Model file for the job. Use its own axes, mm. Face numbers are marked on the shaded views. A direction names the side the tool comes from. Give positions to 0.01 mm unless a question says otherwise; leave off trailing zeros. Write each loop counter-clockwise with the first axis right and the second up, starting at its lowest first coordinate (ties: lowest second). Pieces come first, ordered by that corner, then holes.
```python
from build123d import *

# Parameters (mm, degrees)
F0_W          = 23
F0_H          = 17.5
F1_DEPTH      = 9
F2_T          = -1.2
F3_R          = 5.7
F4_DEPTH      = 3
F3_R_2        = 6.7
F5_DEPTH      = 7.5
F6_W          = 6
F6_H          = 2.3
F6_W_2        = 3.5
F6_H_2        = 3.5
F7_DEPTH      = 4
F8_DEPTH      = 6
F10_DEPTH     = 30
F11_T1_DEPTH  = 19
F11_T3_DEPTH  = 26.5
F11_T5_DEPTH  = 12
F11_T7_DEPTH  = 28.3038475773
F11_S11_W     = 2
F11_S11_H     = 2
F11_T12_DEPTH = 2
F11_S17_W     = 2
F11_S17_H     = 2
F11_T18_DEPTH = 2


# Not quite as in the source:
# - a fillet or chamfer that OpenCascade refuses, or shapes differently, is made with other operations: its cross-section is extruded or revolved along the edge and cut away or added


with BuildPart() as f1:
    # F0 (on Front) → F1 (new body)
    with BuildSketch(Plane.XZ):
        Rectangle(F0_W, F0_H)
    extrude(amount=F1_DEPTH)

    # F2
    f2_openings = [f1.faces().sort_by_distance(p)[0] for p in [
        (0, -9, 0),
    ]]
    offset(amount=F2_T, openings=f2_openings)

    # F3 (on face) → F4 (cut)
    with BuildSketch(Plane(origin=(0, 0, 0), x_dir=(-1, 0, 0), z_dir=(0, 1, 0))):
        Circle(F3_R)
    extrude(amount=-F4_DEPTH, mode=Mode.SUBTRACT)

    # F3 (on face) → F5 (join)
    with BuildSketch(Plane(origin=(0, 0, 0), x_dir=(-1, 0, 0), z_dir=(0, 1, 0))):
        Circle(F3_R_2)
        Circle(F3_R, mode=Mode.SUBTRACT)
    extrude(amount=F5_DEPTH)

    # F6 (on face) → F7 (cut)
    with BuildSketch(Plane.XY.offset(8.75)):
        with Locations((1.5, -7.85)):
            Rectangle(F6_W, F6_H)
        with Locations((-5.75, -7.25)):
            Rectangle(F6_W_2, F6_H_2)
    extrude(amount=-F7_DEPTH, mode=Mode.SUBTRACT)

    # F8 (add): a face of the model
    f8_faces = [f1.faces().sort_by_distance(p)[0] for p in [
        (0, -4.5, -8.75),
    ]]
    extrude(f8_faces, amount=F8_DEPTH)

    # F9 (on face) → F10 (cut)
    with BuildSketch(Plane.YZ.offset(11.5)):
        Polygon((-9, -14.75), (0, -14.75), (-9, -9.5538475773), align=None)
    extrude(amount=-F10_DEPTH, mode=Mode.SUBTRACT)

    # F11: fillet of radius 2 on 7 edges, made by hand

    # F11_s2 → F11_t1 (cut)
    with BuildSketch(Plane.YZ.offset(-9.5)):
        with BuildLine():
            ThreePointArc((0, 6.75), (-0.5857864376, 8.1642135624), (-2, 8.75))
            Line((-2, 8.75), (0, 8.75))
            Line((0, 8.75), (0, 6.75))
        make_face()
    extrude(amount=F11_T1_DEPTH, mode=Mode.SUBTRACT)

    # F11_s4 → F11_t3 (cut)
    with BuildSketch(Plane.XY.offset(-19.75)):
        with BuildLine():
            ThreePointArc((-11.5, -2), (-10.9142135624, -0.5857864376), (-9.5, 0))
            Line((-9.5, 0), (-11.5, 0))
            Line((-11.5, 0), (-11.5, -2))
        make_face()
        with BuildLine():
            ThreePointArc((9.5, 0), (10.9142135624, -0.5857864376), (11.5, -2))
            Line((11.5, -2), (11.5, 0))
            Line((11.5, 0), (9.5, 0))
        make_face()
    extrude(amount=F11_T3_DEPTH, mode=Mode.SUBTRACT)

    # F11_s6 → F11_t5 (cut)
    with BuildSketch(Plane.XZ.offset(2)):
        with BuildLine():
            ThreePointArc((9.5, 8.75), (10.9142135624, 8.1642135624), (11.5, 6.75))
            Line((11.5, 6.75), (11.5, 8.75))
            Line((11.5, 8.75), (9.5, 8.75))
        make_face()
        with BuildLine():
            ThreePointArc((-11.5, 6.75), (-10.9142135624, 8.1642135624), (-9.5, 8.75))
            Line((-9.5, 8.75), (-11.5, 8.75))
            Line((-11.5, 8.75), (-11.5, 6.75))
        make_face()
    extrude(amount=F11_T5_DEPTH, mode=Mode.SUBTRACT)

    # F11_s8 → F11_t7 (cut)
    with BuildSketch(Plane.XY.offset(-14.5538475773)):
        with BuildLine():
            ThreePointArc((-11.5, -7), (-10.9142135624, -8.4142135624), (-9.5, -9))
            Line((-9.5, -9), (-11.5, -9))
            Line((-11.5, -9), (-11.5, -7))
        make_face()
        with BuildLine():
            ThreePointArc((9.5, -9), (10.9142135624, -8.4142135624), (11.5, -7))
            Line((11.5, -7), (11.5, -9))
            Line((11.5, -9), (9.5, -9))
        make_face()
    extrude(amount=F11_T7_DEPTH, mode=Mode.SUBTRACT)


with BuildPart() as f11_tool10:
    # F11_s11 → F11_t12 (new body)
    with BuildSketch(Plane.XZ.offset(2)):
        with Locations((10.5, 7.75)):
            Rectangle(F11_S11_W, F11_S11_H)
    extrude(amount=-F11_T12_DEPTH)

    # F11_s13 → F11_t14 (revolve, cut)
    with BuildSketch(Plane(origin=(9.5, -2, 6.75), x_dir=(-0.7071067812, 0, -0.7071067812), z_dir=(0.7071067812, 0, -0.7071067812))):
        with BuildLine():
            ThreePointArc((0, -2), (2, 0), (0, 2))
            Line((0, 2), (0, -2))
        make_face()
    revolve(axis=Axis((9.5, -2, 6.75), (0, 1, 0)), mode=Mode.SUBTRACT)


with BuildPart() as f1_1:
    add(f1.part)

    # F11_t9: cut F11_tool10
    add(f11_tool10.part, mode=Mode.SUBTRACT)


with BuildPart() as f11_tool16:
    # F11_s17 → F11_t18 (new body)
    with BuildSketch(Plane.YZ.offset(-9.5)):
        with Locations((-1, 7.75)):
            Rectangle(F11_S17_W, F11_S17_H)
    extrude(amount=-F11_T18_DEPTH)

    # F11_s19 → F11_t20 (revolve, cut)
    with BuildSketch(Plane(origin=(-9.5, -2, 6.75), x_dir=(0, -0.7071067812, -0.7071067812), z_dir=(0, 0.7071067812, -0.7071067812))):
        with BuildLine():
            ThreePointArc((0, -2), (2, 0), (0, 2))
            Line((0, 2), (0, -2))
        make_face()
    revolve(axis=Axis((-9.5, -2, 6.75), (-1, 0, 0)), mode=Mode.SUBTRACT)


with BuildPart() as f1_2:
    add(f1_1.part)

    # F11_t15: cut F11_tool16
    add(f11_tool16.part, mode=Mode.SUBTRACT)


solid = f1_2.part
```
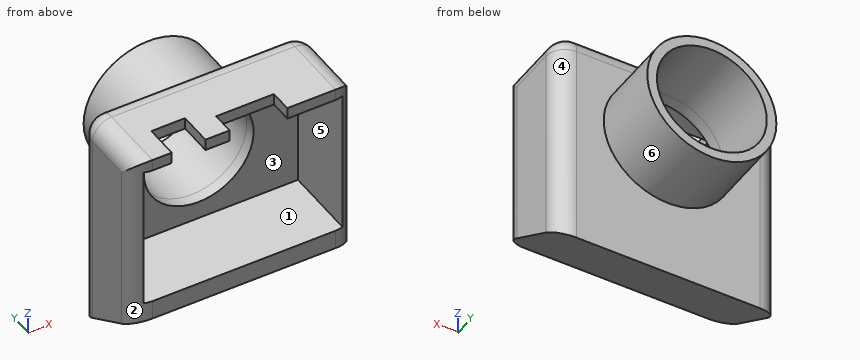
1. Slice it at D-D, the plane x = 8.5. Write the cut outline in (y, z), and give its area (3 significant figures).
Calculated:
outline: (-9, -9.55) - (0, -14.75) - (0, 6.75) arc R2 ccw to (-2, 8.75) - (-9, 8.75) - (-9, 7.55) - (-1.2, 7.55) - (-1.2, -7.55) - (-9, -7.55) - close
area: 69.5 mm2
2. Pull direction Z, two halves, no side cores. Call the marked faces 3, 4, 5 and 6: +Z half, -Z half, draft (parallel to the pull), parting line (faces both ways), or undercut.
Calculated:
face 3: undercut
face 4: draft
face 5: undercut
face 6: parting line
3. Which spindle directions (+Z, -Z, +X, -X, +Y, -Y) get a long thin tool onto all of the face, cutting with end or side? Do the marked faces 1 and 2. Say none if no direction does.
Calculated:
face 1: -Y
face 2: +Z, -Z, -X, -Y
4. Slice it at C-C, the plane y = -7.5. Write the cut outline in (x, z).
Calculated:
outline: (-11.44, -10.42) - (11.44, -10.42) - (11.44, 7.25) arc R2 ccw to (9.5, 8.75) - (4.5, 8.75) - (4.5, 7.55) - (10.3, 7.55) - (10.3, -7.55) - (-10.3, -7.55) - (-10.3, 7.55) - (-7.5, 7.55) - (-7.5, 8.75) - (-9.5, 8.75) arc R2 ccw to (-11.44, 7.25) - close; (-4, 7.55) - (-1.5, 7.55) - (-1.5, 8.75) - (-4, 8.75) - close
5. Slice it at A-A, the plane x = 0. Write the cut outline in (y, z), and give its area (3 significant figures).
Calculated:
outline: (-9, -9.55) - (0, -14.75) - (0, -6.7) - (7.5, -6.7) - (7.5, -5.7) - (-1.2, -5.7) - (-1.2, -7.55) - (-9, -7.55) - close; (-6.7, 7.55) - (-1.2, 7.55) - (-1.2, 5.7) - (7.5, 5.7) - (7.5, 6.7) - (0, 6.7) - (0, 6.75) arc R2 ccw to (-2, 8.75) - (-6.7, 8.75) - close
area: 68.0 mm2
6. Probe probe 1 along X at (y, z) = (-5.5, -1); probe 2 along Y at (x, z) = (1.25, -6.75); probe 3 along X at (y, z) = (-7.75, -6). List the from-to ranges inside material, lowest first.
Calculated:
probe 1: x = -11.5 to -10.3, 10.3 to 11.5
probe 2: y = -1.2 to 0
probe 3: x = -11.35 to -10.3, 10.3 to 11.35
7. Pin check, flat tips, straight feed: P1, Ø1.3, axis at y = -6.5, z = 8, coming from the -X side; P2, Ø1.3, axis at y = -8, z = 8, coming from the +X side; P3, Ø1, axis at y = 1, z = 0.5, coming from the -X side. Stop position of each tip, or through.
Calculated:
P1: stops at x = -11.41
P2: stops at x = 11.38
P3: stops at x = -6.7
8. Slice it at B-B, the plane z = 0. Write the cut outline in (x, y), and give its area (3 significant figures).
Calculated:
outline: (-11.5, -7) arc R2 ccw to (-10.3, -8.83) - (-10.3, -1.2) - (-5.7, -1.2) - (-5.7, 7.5) - (-6.7, 7.5) - (-6.7, 0) - (-9.5, 0) arc R2 ccw to (-11.5, -2) - close; (5.7, -1.2) - (10.3, -1.2) - (10.3, -8.83) arc R2 ccw to (11.5, -7) - (11.5, -2) arc R2 ccw to (9.5, 0) - (6.7, 0) - (6.7, 7.5) - (5.7, 7.5) - close
area: 44.3 mm2
